Could you check a few things on this model? Use its own coordinates, in mm. Coordinates: 2 decimals unless noted, no trailing zeros. Write each loop counter-clockwise with the first axis right and the second up, starting at its lowest first coordinate (ties: lowest second). Pieces come first, ordered by that corner, then holes. Notation, with made-up numbers: M 67.25,10.5 L 108.25,10.5 A17 cw 108.25,23.5 Z; hole C 40.25,8 d5. An arc over 180 degrees is marked long. Answer as CSV lines item,"result". Start each with the question number.
Item 1: I'm going to push flat-ended pins straight in: P1, Ø12, axis at x = -22, y = -14.5, coming from the +Z side; P2, Ø6, axis at y = -7, z = -43.5, coming from the -X side; P3, Ø1, axis at y = -11, z = -31, coming from the +X side. Where does each tip first touch, or does it pass through?
Item 2: Suppose I cut it at A-A, the plane z = 0. Write out the boundary of the cut face in (x, y).
Item 3: Suppose I cut it at C-C, the plane y = -14. Write out the boundary of the cut face in (x, z).
Item 4: If I drill on line 1 along Z through (x, y) = (0, -1); line 2 along Z through (x, y) = (-1, 10); line 3 along X through (y, z) = (-3, 3), over which ranges is the centre line in solid material (lowest first)? Write a range as [from, to].
Item 5: Suppose I cut it at D-D, the plane y = 3. Write out the boundary of the cut face in (x, z).
Item 6: Suppose I cut it at B-B, the plane x = 0. Write out the boundary of the cut face in (y, z), and give its area (3 significant figures).
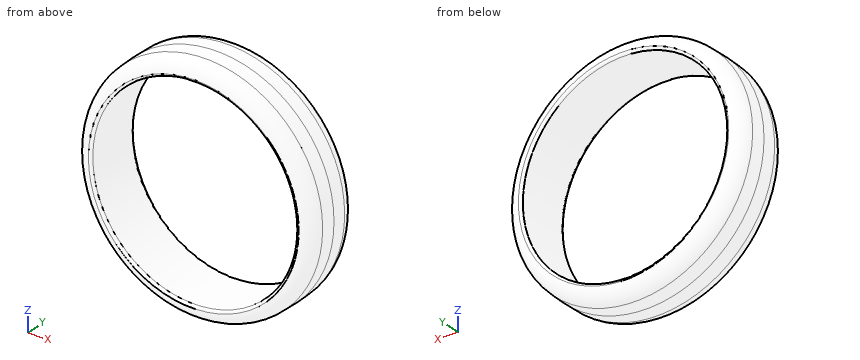
Autodesk Inventor part; units mm, degrees
ref_plane "YZ Plane" through (0, 0, 0) normal (1, 0, 0) x (0, 1, 0)
ref_plane "XZ Plane" through (0, 0, 0) normal (0, 1, 0) x (-1, 0, 0)
ref_plane "XY Plane" through (0, 0, 0) normal (0, 0, 1) x (1, 0, 0)
sketch "Sketch1" plane through (0, 0, 0) normal (0, 0, 1) x (1, 0, 0)
  line L0 (-66.6603, -11.4443) -> (-66.6119, -11.4443)
  arc A0 (-68.3474, -19.0449) -> (-66.633, -17.4625) centre (-68.2205, -17.4625) ccw
  arc A1 (-77.1082, -9.779) -> (-68.3474, -19.0449) centre (-67.586, -9.5504) ccw
  line L1 (-77.1082, -9.779) -> (-77.343, 0)
  line L2 (-77.343, 0) -> (-77.1082, 9.779)
  arc A2 (-68.3474, 19.0449) -> (-77.1082, 9.779) centre (-67.586, 9.5504) ccw
  arc A3 (-66.633, 17.4625) -> (-68.3474, 19.0449) centre (-68.2205, 17.4625) ccw
  line L3 (-66.633, 17.4625) -> (-66.633, -17.4625)
  line L4 (0, -29.0182) -> (0, 29.0182)
  point P0 (0, 0)
  point P1 (-66.633, 0)
  dimension "d0" = 38.1
  dimension "d1" = 1.5875
  dimension "d2" = 9.525
  dimension "d3" = 19.558
  dimension "d10" = 77.343
revolve "Revolution1" add sketch "Sketch1" angle 360 about axis through (0, -10, 0) along (0, 1, 0)
properties part number "First 09 Wheel_6+375 tread Simple"
Ans:
1,P1,"stops at z = 75.07"
1,P2,"stops at x = -65.7"
1,P3,"stops at x = 70.72"
2,outline,"M -77.34,0 L -77.11,-9.78 A9.53 ccw -68.35,-19.04 A1.59 ccw -66.63,-17.46 L -66.63,17.46 A1.59 ccw -68.35,19.04 A9.52 ccw -77.11,9.78 Z; M 66.63,-17.46 A1.59 ccw 68.35,-19.04 A9.53 ccw 77.11,-9.78 L 77.34,0 L 77.11,9.78 A9.52 ccw 68.35,19.04 A1.59 ccw 66.63,17.46 Z"
3,outline,"C 0,0 d152.02; hole C 0,0 d133.27"
4,line 1,"z = [-77.32, -66.63], [66.63, 77.32]"
4,line 2,"z = [-77.09, -66.63], [66.63, 77.09]"
4,line 3,"x = [-77.21, -66.57], [66.57, 77.21]"
5,outline,"C 0,0 d154.54; hole C 0,0 d133.27"
6,outline,"M -19.04,-68.35 A9.53 ccw -9.78,-77.11 L 0,-77.34 L 9.78,-77.11 A9.52 ccw 19.04,-68.35 A1.59 ccw 17.46,-66.63 L -17.46,-66.63 A1.59 ccw Z; M -19.04,68.35 A1.59 ccw -17.46,66.63 L 17.46,66.63 A1.59 ccw 19.04,68.35 A9.52 ccw 9.78,77.11 L 0,77.34 L -9.78,77.11 A9.53 ccw Z"
6,area,"724 mm^2"
